```python
from build123d import *

# Parameters (mm, degrees)
F1_DEPTH = 254
F2_R     = 3.175
F3_DEPTH = 25.4


with BuildPart() as f1:
    # F0 (on Front) → F1 (new body)
    with BuildSketch(Plane.XZ):
        Polygon((-17.78, 0), (0, 0), (0, 19.05), (-5.08, 19.05), (-5.08, 5.08), (-17.78, 5.08), align=None)
    extrude(amount=F1_DEPTH)

    # F2 (on face) → F3 (cut)
    with BuildSketch(Plane.YZ):
        with Locations((-241.3, 13.209414)):
            Circle(F2_R)
        with Locations((-114.3, 12.615733)):
            Circle(F2_R)
    extrude(amount=-F3_DEPTH, mode=Mode.SUBTRACT)


solid = f1.part
```
CAD build for the part. Positions are in the model's coordinates, mm. A direction names the side the tool comes from. Coordinates: 2 decimals unless noted, no trailing zeros. Order: outer loops, then holes, each group sorted by start corner. A loop starts at its lowest first (then second) coordinate and runs counter-clockwise, first axis right, second up. Notation, with made-up numbers: M 29,-22 L 38,-22 A23 ccw 38,10 Z; hole C 33.25,34 d2. An arc over 180 degrees is marked long. Write each question's results on one line, items separated by ' | '. Start each with the question number.
Q1. Flat gauge pins, fed straight in: P1, Ø4, axis at x = -15, y = -35, coming from the +Z side; P2, Ø11, axis at y = -152, z = 13, coming from the -X side. Where does each tip first touch, or does it go through?
Q2. Which spindle directions (+Z, -Z, +X, -X, +Y, -Y) get a long thin tool onto all of the face, cutting with end or side? Do faces 1 (the flat face through (-5.08, -125, 12)), 2 (the flat face through (-3, -254, 8)). Say none if no direction does.
Q3. Pull direction Z, two halves, no side cores. Call faces 3 (the flat face through (-3, -125, 19.05)), 4 (the cylindrical face through (-2.5, -117.47, 12.76)), 5 (the flat face through (-17.78, -125, 3)): +Z half, -Z half, draft (parallel to the pull), parting line (faces both ways), or undercut.
Q4. Drill centre lines: probe 1 along Y at (x, z) = (-1.5, 12.75); probe 2 along Z at (x, y) = (-3.3, -114.3); probe 3 along Z at (x, y) = (-8, -131). Where is each one in solid material? Low to high. Write a range as from..to.
Q5. Cut at B-B (x = -8). List the corners of the cut face in (y, z).
Q6. Cut at A-A (y = -114.3). List the corners of the cut face in (x, z), then the cut area to 3 significant figures.
Found:
1) P1: z = 5.08 | P2: x = -5.08
2) face 1: +Z, -X, +Y, -Y | face 2: +Z, -Z, +X, -X, -Y
3) face 3: +Z half | face 4: undercut | face 5: draft
4) probe 1: -254..-244.44, -238.16..-117.47, -111.13..0 | probe 2: 0..9.44, 15.79..19.05 | probe 3: 0..5.08
5) outline: M -254,0 L 0,0 L 0,5.08 L -254,5.08 Z
6) outline: M -17.78,0 L 0,0 L 0,9.44 L -5.08,9.44 L -5.08,5.08 L -17.78,5.08 Z; M -5.08,15.79 L 0,15.79 L 0,19.05 L -5.08,19.05 Z | area: 129 mm²
